The model under review builds one solid part; all positions refer to its coordinate system, in mm. Face numbers are marked on the shaded views. A direction names the side the tool comes from. Round coordinates to 2 decimals unless told otherwise and drop trailing zeros. Loops run counter-clockwise (first coordinate to the right, second up) from the corner with the lowest first, then second, coordinate; pieces in that order, holes last. Notation, with made-up numbers: M 7,-9 L 59,-9 A7 ccw 59,2 Z; hole C 87,68.25 d5. An arc over 180 degrees is marked long. Return JSON: item names as keys, results as strings. Group by question number.
Q1. Consider section D-D (z = -24.5). State the section outline as (x, y) points.
Q2. For the marked faces 1 and 2, list the 3-axis set-ups (+Z, -Z, +X, -X, +Y, -Y) from which the entire face can be reached by the end or side of a thin tool; tool diameter is ignored.
Q3. Consider section A-A (y = 0). State the section outline as (x, z) points, and give its area (3 significant figures).
Q4. Consider section B-B (z = 25). State the section outline as (x, y) points, and give its area (3 significant figures).
Q5. Draft analysis for pull direction Y (two halves, no side actions). For the marked faces 3, 4 and 5, state which applies: pulls with the +Y half, pulls with the -Y half, needs draft (parallel to the pull), parting line crosses it, or undercut.
Q6. Clearance check with flat-ended pins moving along their axes: pin 1 Ø6 at (x, z) = (-9.5, 17) entering from +Y; pin 2 Ø2 at (y, z) = (-2.5, 22.5) entering from +X; pin 3 Ø1 at (x, z) = (-31, -37) entering from +Y. State where each tip first meets the part, or that it passes through.
Q7. To check wall thickness, follow line 1 along X through (y, z) = (1, 18.5); line 2 along X through (y, z) = (-4.5, 25). State the ranges of each line that lie inside material, in increasing order.
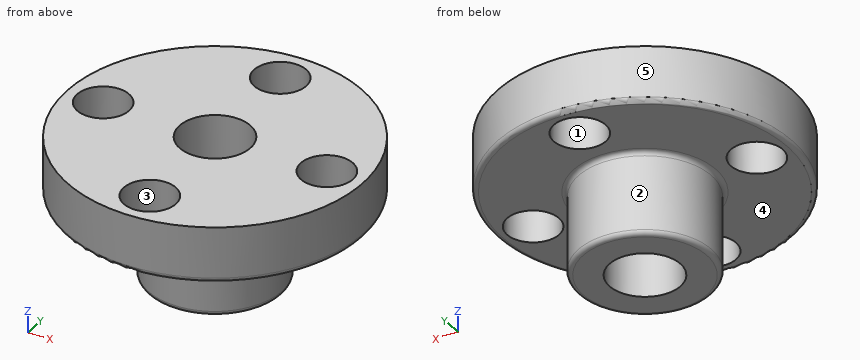
from build123d import *

# Parameters (mm, degrees)
SKETCH1_R           = 80.562529646
BOSS_EXTRUDE1_DEPTH = 30.48
SKETCH3_R           = 36.406797413
BOSS_EXTRUDE2_DEPTH = 45.72
SKETCH4_R           = 19.383893348
CUT_EXTRUDE1_DEPTH  = 138.065978148
SKETCH5_R           = 14.222468522
CUT_EXTRUDE2_DEPTH  = 122.840694211
CIRPATTERN2_COUNT   = 4
FILLET1_R           = 2.54
FILLET2_R           = 2.54


with BuildPart() as part:
    # Sketch1 → Boss-Extrude1 (new body)
    with BuildSketch(Plane.XY):
        with Locations(Location((0, 0, 0), (0, 0, 180))):
            Circle(SKETCH1_R)
    extrude(amount=BOSS_EXTRUDE1_DEPTH)

    # Sketch3 → Boss-Extrude2 (add)
    with BuildSketch(Plane(origin=(0, 0, 0), x_dir=(-1, 0, 0), z_dir=(0, 0, -1))):
        with Locations(Location((0, 0, 0), (0, 0, 180))):
            Circle(SKETCH3_R)
    extrude(amount=BOSS_EXTRUDE2_DEPTH)

    # Sketch4 → Cut-Extrude1 (cut, through all)
    with BuildSketch(Plane(origin=(0, 0, -45.72), x_dir=(-1, 0, 0), z_dir=(0, 0, -1))):
        Circle(SKETCH4_R)
    extrude(amount=-CUT_EXTRUDE1_DEPTH, mode=Mode.SUBTRACT)

    # Sketch5 → Cut-Extrude2 (cut, through all)
    with BuildSketch(Plane(origin=(0, 0, -2.54), x_dir=(-1, 0, 0), z_dir=(0, 0, -1))):
        with Locations((-60.632628963, 0)):
            Circle(SKETCH5_R)
    cut_extrude2 = extrude(amount=-CUT_EXTRUDE2_DEPTH, mode=Mode.SUBTRACT)

    # CirPattern2: Cut-Extrude2 ×4 about axis
    cirpattern2_axis = Axis((0, 0, 0), (0, 0, 1))
    for i in range(1, CIRPATTERN2_COUNT):
        add(cut_extrude2.rotate(cirpattern2_axis, i * 360 / CIRPATTERN2_COUNT), mode=Mode.SUBTRACT)

    # Fillet1
    fillet1_edges = [part.edges().sort_by_distance(p)[0] for p in [
        (-36.406797413, 0, 0),
        (-36.406797413, 0, -45.72),
    ]]
    fillet(fillet1_edges, radius=FILLET1_R)

    # Fillet2
    fillet2_edges = [part.edges().sort_by_distance(p)[0] for p in [
        (80.562529646, 0, 0),
    ]]
    fillet(fillet2_edges, radius=FILLET2_R)


solid = part.part
Values:
{
 "1": {"outline": "C 0,0 d72.81; hole C 0,0 d38.77"},
 "2": {"face 1": "+Z, -Z", "face 2": "-Z"},
 "3": {"outline": "M -80.56,2.54 A2.54 ccw -78.02,0 L -74.86,0 L -74.86,30.48 L -80.56,30.48 Z; M -46.41,0 L -38.95,0 A2.54 cw -36.41,-2.54 L -36.41,-43.18 A2.54 ccw -33.87,-45.72 L -19.38,-45.72 L -19.38,30.48 L -46.41,30.48 Z; M 19.38,-45.72 L 33.87,-45.72 A2.54 ccw 36.41,-43.18 L 36.41,-2.54 A2.54 cw 38.95,0 L 46.41,0 L 46.41,30.48 L 19.38,30.48 Z; M 74.86,0 L 78.02,0 A2.54 ccw 80.56,2.54 L 80.56,30.48 L 74.86,30.48 Z", "area": "3,550 mm2"},
 "4": {"outline": "C 0,0 d161.13; hole C -60.63,0 d28.44; hole C 0,0 d38.77; hole C 0,-60.63 d28.44; hole C 0,60.63 d28.44; hole C 60.63,0 d28.44", "area": "16,700 mm2"},
 "5": {"face 3": "undercut", "face 4": "needs draft", "face 5": "parting line crosses it"},
 "6": {"pin 1": "stops at y = 80.3", "pin 2": "stops at x = 80.55", "pin 3": "stops at y = 19.88"},
 "7": {"line 1": "x = -80.56 to -74.82, -46.45 to -19.36, 19.36 to 46.45, 74.82 to 80.56", "line 2": "x = -80.44 to -74.12, -47.14 to -18.85, 18.85 to 47.14, 74.12 to 80.44"}
}
